```python
from build123d import *

# Parameters (mm, degrees)
SKETCH1_R                                            = 18
SKETCH1_R_2                                          = 6.2
BOSS_EXTRUDE1_DEPTH                                  = 3
BOSS_EXTRUDE2_START                                  = -5
SKETCH5_R                                            = 20
SKETCH5_R_2                                          = 18
BOSS_EXTRUDE2_DEPTH                                  = 5
BOSS_EXTRUDE3_START                                  = -5
BOSS_EXTRUDE3_DEPTH                                  = 5
SKETCH7_W                                            = 40
SKETCH7_H                                            = 45
BOSS_EXTRUDE4_DEPTH                                  = 6
SKETCH8_W                                            = 46
SKETCH8_H                                            = 14
BOSS_EXTRUDE5_DEPTH                                  = 6
BOSS_EXTRUDE6_DEPTH                                  = 6
CHAMFER1_SIZE                                        = 8
CSK_FOR_M3_HEX_SOCKET_COUNTERSUNK_HEAD_S_D           = 3.6
CSK_FOR_M3_HEX_SOCKET_COUNTERSUNK_HEAD_S_CSINK_D     = 6.94
CSK_FOR_M3_HEX_SOCKET_COUNTERSUNK_HEAD_S_CSINK_ANGLE = 90
BOSS_EXTRUDE7_DEPTH                                  = 5
M3_CLEARANCE_HOLE3_D                                 = 3.6
SKETCH26_R                                           = 4.25
CUT_EXTRUDE3_DEPTH                                   = 2


with BuildPart() as part:
    # Sketch1 → Boss-Extrude1 (new body)
    with BuildSketch(Plane(origin=(0, 0, 0), x_dir=(1, 0, 0), z_dir=(0, 1, 0))):
        with Locations(Location((0, 0, 0), (0, 0, 270))):
            Circle(SKETCH1_R)
        with Locations(Location((0, 0, 0), (0, 0, 270))):
            Circle(SKETCH1_R_2, mode=Mode.SUBTRACT)
    extrude(amount=BOSS_EXTRUDE1_DEPTH)

    # Sketch5 → Boss-Extrude2 (add)
    with BuildSketch(Plane(origin=(0, 3, 0), x_dir=(1, 0, 0), z_dir=(0, 1, 0)).offset(BOSS_EXTRUDE2_START)):
        with Locations(Location((0, 0, 0), (0, 0, 270))):
            Circle(SKETCH5_R)
        with Locations(Location((0, 0, 0), (0, 0, 270))):
            Circle(SKETCH5_R_2, mode=Mode.SUBTRACT)
    extrude(amount=BOSS_EXTRUDE2_DEPTH)

    # Sketch6 → Boss-Extrude3 (add)
    with BuildSketch(Plane(origin=(0, 3, 0), x_dir=(1, 0, 0), z_dir=(0, 1, 0)).offset(BOSS_EXTRUDE3_START)):
        with BuildLine():
            Line((-20, 0), (-20, -31))
            Line((-20, -31), (20, -31))
            Line((20, -31), (20, 0))
            ThreePointArc((20, 0), (0, -20), (-20, 0))
        make_face()
    extrude(amount=BOSS_EXTRUDE3_DEPTH)

    # Sketch7 → Boss-Extrude4 (add)
    with BuildSketch(Plane.XY.offset(31)):
        with Locations((0, 20.5)):
            Rectangle(SKETCH7_W, SKETCH7_H)
    extrude(amount=BOSS_EXTRUDE4_DEPTH)

    # Sketch8 → Boss-Extrude5 (add)
    with BuildSketch(Plane.XY.offset(37)):
        with Locations((0, 36)):
            Rectangle(SKETCH8_W, SKETCH8_H)
    extrude(amount=-BOSS_EXTRUDE5_DEPTH)

    # Sketch9 → Boss-Extrude6 (add)
    with BuildSketch(Plane.XY.offset(37)):
        Polygon((-23, 29), (-20, -2), (-20, 29), align=None)
        Polygon((20, -2), (23, 29), (20, 29), align=None)
    extrude(amount=-BOSS_EXTRUDE6_DEPTH)

    # Chamfer1
    chamfer1_edges = [part.edges().sort_by_distance(p)[0] for p in [
        (0, 3, 31),
    ]]
    chamfer(chamfer1_edges, length=CHAMFER1_SIZE)

    # CSK for M3 Hex Socket Countersunk Head Screw1 (through all)
    with Locations(Plane.XY.offset(37)):
        with Locations((17.5, 36.752814471), (-17.5, 36.752814471)):
            CounterSinkHole(CSK_FOR_M3_HEX_SOCKET_COUNTERSUNK_HEAD_S_D / 2, CSK_FOR_M3_HEX_SOCKET_COUNTERSUNK_HEAD_S_CSINK_D / 2, counter_sink_angle=CSK_FOR_M3_HEX_SOCKET_COUNTERSUNK_HEAD_S_CSINK_ANGLE)

    # Sketch23 → Boss-Extrude7 (add)
    with BuildSketch(Plane.XZ.offset(2)):
        with BuildLine():
            Line((0, -20), (32, -20))
            Line((32, -20), (32, 18))
            Line((32, 18), (20, 18))
            Line((20, 18), (20, 0))
            ThreePointArc((20, 0), (14.142135624, -14.142135624), (0, -20))
        make_face()
    extrude(amount=-BOSS_EXTRUDE7_DEPTH)

    # M3 Clearance Hole3 (through all)
    with Locations(Plane(origin=(0, -2, 0), x_dir=(-1, 0, 0), z_dir=(0, -1, 0))):
        with Locations((-24.8, 9.35), (8.9, 9.35), (8.9, -9.35), (-24.8, -9.35)):
            Hole(M3_CLEARANCE_HOLE3_D / 2)

    # Sketch26 → Cut-Extrude3 (cut)
    with BuildSketch(Plane.XZ.offset(2)):
        with Locations(Location((24.8, 9.35, 0), (0, 0, 270))):
            Circle(SKETCH26_R)
        with Locations(Location((24.8, -9.35, 0), (0, 0, 270))):
            Circle(SKETCH26_R)
    extrude(amount=-CUT_EXTRUDE3_DEPTH, mode=Mode.SUBTRACT)


solid = part.part
```
Design review of the part built by this model. Coordinates are the model's own, in mm. A direction names the side the tool comes from. Coordinates: 2 decimals unless noted, no trailing zeros. Loops run counter-clockwise (first coordinate to the right, second up) from the corner with the lowest first, then second, coordinate; pieces in that order, holes last. Notation, with made-up numbers: (-30, -30) -> (22, -30) arc R28 ccw to (22, -10) -> close; hole circle Ø2 at (54, -28). An arc over 180 degrees is marked (long way). Answer as a JSON object with one key per item and string values.
Q1. Take a section at B-B on x = 4. Give the boundary of the cut face in (y, z).
Answer block:
{"outline": "(-2, -20) -> (3, -20) -> (3, -4.74) -> (0, -4.74) -> (0, -17.55) -> (-2, -17.55) -> close; (-2, 17.55) -> (0, 17.55) -> (0, 4.74) -> (3, 4.74) -> (3, 23) -> (11, 31) -> (43, 31) -> (43, 37) -> (-2, 37) -> close"}
Q2. Tool access review of faces 4 (the flat face through (21.48, 13.28, 34.04)), 5 (the flat face through (6, 3, 7)), 6 (the cylindrical face through (5.407, -1.014, 17.169)): name each direction out of +Z, -Z, +X, -X, +Y, -Y from which nothing blocks a thin tool from reaching the whole face with its end or side.
Answer block:
{"face 4": "+Z, +X, -Y", "face 5": "-Z, +X, -X, +Y", "face 6": "-Y"}
Q3. Take a section at D-D on z = 9.35. Give the boundary of the cut face in (x, y).
Answer block:
{"outline": "(-20, -2) -> (-15.38, -2) -> (-15.38, 0) -> (-10.7, 0) -> (-10.7, 3) -> (-20, 3) -> close; (-7.1, 0) -> (15.38, 0) -> (15.38, -2) -> (20.55, -2) -> (20.55, 0) -> (23, 0) -> (23, 3) -> (-7.1, 3) -> close; (26.6, 0) -> (29.05, 0) -> (29.05, -2) -> (32, -2) -> (32, 3) -> (26.6, 3) -> close"}
Q4. Take a section at A-A on z = -4. Give the boundary of the cut face in (x, y), plus the area to 3 significant figures.
Answer block:
{"outline": "(-19.6, -2) -> (-17.55, -2) -> (-17.55, 0) -> (-4.74, 0) -> (-4.74, 3) -> (-19.6, 3) -> close; (4.74, 0) -> (17.55, 0) -> (17.55, -2) -> (32, -2) -> (32, 3) -> (4.74, 3) -> close", "area": "159 mm^2"}
Q5. To check wall thickness, follow L1, parallel to Z at x = 24.8, y = 2; L2, parallel to X at y = 1.45, z = 9.35; L3, parallel to X at y = -1.2, z = -9.35. State the ranges of each line that lie inside material, in increasing order.
Answer block:
{"L1": "z = -20 to -11.15, -7.55 to 7.55, 11.15 to 18", "L2": "x = -20 to -10.7, -7.1 to 23, 26.6 to 32", "L3": "x = -17.68 to -15.38, 15.38 to 20.55, 29.05 to 32"}
Q6. Take a section at C-C on x = 24.8. Give the boundary of the cut face in (y, z).
Answer block:
{"outline": "(-2, -20) -> (3, -20) -> (3, -11.15) -> (0, -11.15) -> (0, -13.6) -> (-2, -13.6) -> close; (-2, -5.1) -> (0, -5.1) -> (0, -7.55) -> (3, -7.55) -> (3, 7.55) -> (0, 7.55) -> (0, 5.1) -> (-2, 5.1) -> close; (-2, 13.6) -> (0, 13.6) -> (0, 11.15) -> (3, 11.15) -> (3, 18) -> (-2, 18) -> close"}
Q7. The part is to be moulded in two halves that separate along Z. For faces 1 (the cylindrical face through (-13.986, 0.465, -14.297)), 2 (the flat face through (-20, 2, 15)), 3 (the flat face through (23, 0, -10.2)), say which applies: +Z half, -Z half, draft (parallel to the pull), parting line (faces both ways), or undercut.
Answer block:
{"face 1": "-Z half", "face 2": "draft", "face 3": "undercut"}
Q8. Clearance check with flat-ended pins moving along their axes: pin 1 Ø3 at (y, z) = (39, 32.5) entering from +X; pin 2 Ø1.5 at (x, z) = (-6.5, 22) entering from +Y; pin 3 Ø5.5 at (x, y) = (24, 1) entering from +Z; pin 4 Ø7.5 at (x, z) = (0, 0) entering from -Y. State where each tip first meets the part, or that it passes through.
Answer block:
{"pin 1": "stops at x = 23", "pin 2": "stops at y = 3", "pin 3": "stops at z = 18", "pin 4": "passes through"}
